```python
from build123d import *

# Parameters (mm, degrees)
SKETCH1_R           = 2.125
SKETCH1_R_2         = 4.025
BOSS_EXTRUDE1_DEPTH = 2.5
FILLET1_R           = 4


with BuildPart() as part:
    # Sketch1 → Boss-Extrude1 (new body, symmetric)
    with BuildSketch(Plane(origin=(0, 0, 0), x_dir=(1, 0, 0), z_dir=(0, 1, 0))):
        Polygon((-57.5, 30), (-57.5, -5), (-72.5, -5), (-72.5, 30), (-41.660750149, 58.750444357), (-26.660750149, 58.750444357), align=None)
        with Locations((-65, 25)):
            Circle(SKETCH1_R, mode=Mode.SUBTRACT)
        with Locations((-65, 15)):
            Circle(SKETCH1_R, mode=Mode.SUBTRACT)
        with Locations((-42.584679142, 50.750444357)):
            Circle(SKETCH1_R_2, mode=Mode.SUBTRACT)
        with Locations((-65, 5)):
            Circle(SKETCH1_R, mode=Mode.SUBTRACT)
    extrude(amount=BOSS_EXTRUDE1_DEPTH, both=True)

    # Fillet1
    fillet1_edges = [part.edges().sort_by_distance(p)[0] for p in [
        (-72.5, 0, -30),
        (-41.660750149, 0, -58.750444357),
        (-26.660750149, 0, -58.750444357),
        (-57.5, 0, -30),
    ]]
    fillet(fillet1_edges, radius=FILLET1_R)


solid = part.part
```
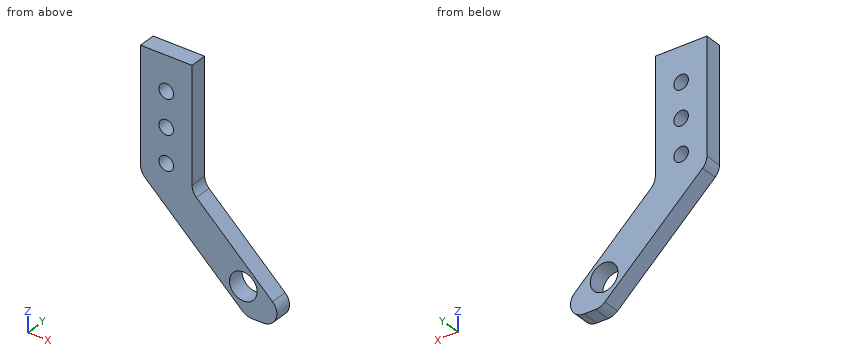
Model file for the job. Use its own axes, mm. Coordinates: 2 decimals unless noted, no trailing zeros. Order: outer loops, then holes, each group sorted by start corner. A loop starts at its lowest first (then second) coordinate and runs counter-clockwise, first axis right, second up. Notation, with made-up numbers: (30, 36) -> (44, 36) arc R28 cw to (44, 60) -> close; hole circle Ø8 at (54.25, 67). An arc over 180 degrees is marked (long way). Answer as a JSON object with one key per item and string values. Group by question number.
1) Cut at B-B, the plane x = -41. Write the cut outline in (y, z).
2) Drill centre lines: L1, parallel to X at y = 1.25, z = -5 (3 decimals); L2, parallel to Z at x = -64.5, y = -0.25; L3, parallel to X at y = 2, z = -8.5. Where is each one in solid material? Low to high.
3) Cut at A-A, the plane z = -25. Write the cut outline in (x, y) (3 decimals), then the cut area to 4 significant figures.
4) Cut at D-D, the plane y = -0.9. Write the cut outline in (x, z) (3 decimals).
5) Cut at C-C, the plane x = -64. Write the cut outline in (y, z) (3 decimals).
6) Flat gauge pins, fed straight in: pin 1 (5 mm diameter, centred on x = -42.58, z = -50.75, fed in from -Y); pin 2 (3 mm diameter, centred on x = -43, y = 2, fed in from -Z). Where does each tip first touch, or does it go through?
Check values:
{
 "1": {"outline": "(-2.5, -58.64) -> (2.5, -58.64) -> (2.5, -54.45) -> (-2.5, -54.45) -> close; (-2.5, -47.05) -> (2.5, -47.05) -> (2.5, -45.38) -> (-2.5, -45.38) -> close"},
 "2": {"L1": "x = -72.5 to -67.125, -62.875 to -57.5", "L2": "z = -37.46 to -27.07, -22.93 to -17.07, -12.93 to -7.07, -2.93 to 5", "L3": "x = -72.5 to -57.5"},
 "3": {"outline": "(-72.5, -2.5) -> (-67.125, -2.5) -> (-67.125, 2.5) -> (-72.5, 2.5) -> close; (-62.875, -2.5) -> (-57.5, -2.5) -> (-57.5, 2.5) -> (-62.875, 2.5) -> close", "area": "53.75 mm²"},
 "4": {"outline": "(-72.5, -28.26) arc R4 ccw to (-71.228, -31.186) -> (-42.813, -57.676) arc R4 ccw to (-40.085, -58.75) -> (-36.817, -58.75) arc R4 ccw to (-34.09, -51.825) -> (-56.228, -31.186) arc R4 cw to (-57.5, -28.26) -> (-57.5, 5) -> (-72.5, 5) -> close; hole circle Ø4.25 at (-65, -25); hole circle Ø4.25 at (-65, -15); hole circle Ø4.25 at (-65, -5); hole circle Ø8.05 at (-42.585, -50.75)"},
 "5": {"outline": "(-2.5, -37.924) -> (2.5, -37.924) -> (2.5, -26.875) -> (-2.5, -26.875) -> close; (-2.5, -23.125) -> (2.5, -23.125) -> (2.5, -16.875) -> (-2.5, -16.875) -> close; (-2.5, -13.125) -> (2.5, -13.125) -> (2.5, -6.875) -> (-2.5, -6.875) -> close; (-2.5, -3.125) -> (2.5, -3.125) -> (2.5, 5) -> (-2.5, 5) -> close"},
 "6": {"pin 1": "passes through", "pin 2": "stops at z = -58.49"}
}
